Could you check a few things on this model? Use its own coordinates, in mm. Give positions to 0.01 mm unless a question says otherwise; leave off trailing zeros. Order: outer loops, then holes, each group sorted by start corner. A loop starts at its lowest first (then second) coordinate and runs counter-clockwise, first axis right, second up. Notation, with made-up numbers: M -22,4.25 L 37,4.25 A21 cw 37,29.25 Z; hole C -8,73 d2. An arc over 180 degrees is marked long. Return JSON: item names as keys, results as strings. Group by question number.
```python
from build123d import *

# Parameters (mm, degrees)
EXTRUDE_1_DEPTH            = 3.2
FILLET_1_R                 = 5
SKETCH_2_R                 = 2.1
CUT_EXTRUDE_1_DEPTH        = 3.2
PATTERN_LINEAR_1_COUNT     = 2
PATTERN_LINEAR_1_PITCH     = 45
PATTERN_LINEAR_1_COL_COUNT = 2
PATTERN_LINEAR_1_COL_PITCH = 45


with BuildPart() as part:
    # Эскиз1 → Бобышка-Вытянуть1 (new body)
    with BuildSketch(Plane.XY):
        Polygon((0, 0), (150, 0), (180, 220), (130, 220), align=None)
    extrude(amount=EXTRUDE_1_DEPTH)

    # Скругление1
    fillet_1_edges = [part.edges().sort_by_distance(p)[0] for p in [
        (130, 220, 1.6),
        (180, 220, 1.6),
        (150, 0, 1.6),
        (0, 0, 1.6),
    ]]
    fillet(fillet_1_edges, radius=FILLET_1_R)

    # Эскиз2 → Вырез-Вытянуть1 (cut)
    with BuildSketch(Plane.XY.offset(3.2)):
        with Locations((77.198893337, 10)):
            Circle(SKETCH_2_R)
    cut_extrude_1 = extrude(amount=-CUT_EXTRUDE_1_DEPTH, mode=Mode.SUBTRACT)

    # Линейный массив1: Вырез-Вытянуть1 ×2
    with Locations(*[(i * PATTERN_LINEAR_1_PITCH, 0, 0) for i in range(1, PATTERN_LINEAR_1_COUNT)]):
        add(cut_extrude_1, mode=Mode.SUBTRACT)

    # Линейный массив1 col: Вырез-Вытянуть1 ×2
    with Locations(*[(-i * PATTERN_LINEAR_1_COL_PITCH, 0, 0) for i in range(1, PATTERN_LINEAR_1_COL_COUNT)]):
        add(cut_extrude_1, mode=Mode.SUBTRACT)


solid = part.part
```
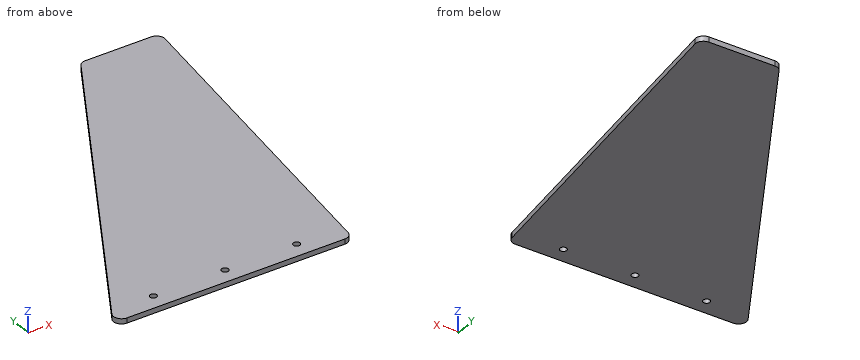
1. Imagine slicing it at A-A, the plane z = 1.8. Please give me the cut outline in (x, y), plus the area to 3 significant figures.
2. Imagine slicing it at B-B, the plane x = 65.5. Please give me the cut outline in (y, z), plus the area to 3 significant figures.
3. For pin 1 (2.5 mm diameter, centred on x = 77.2, y = 10, fed in from +Z); pin 2 (1 mm diameter, centred on x = 98, y = 57.5, fed in from -Z); pin 3 (1 mm diameter, centred on y = 144, z = 2, fed in from -X), each with a flat end and sliding along its axis, tell me the tip position at first contact or that it passes through.
4. Imagine slicing it at C-C, the plane y = 118. Please give me the cut outline in (x, z), plus the area to 3 significant figures.
5. I need wall thicknesses on L1, parallel to Y at x = 146, z = 0.9; L2, parallel to X at y = 138.5, z = 0.5; L3, parallel to Y at x = 53, z = 2.3. Which ranges of each line are inside material? Lowest first, please. Write a range as from..to.
Values:
{
 "1": {"outline": "M 4.46,7.54 A5 ccw 8.76,0 L 145.64,0 A5 ccw 150.59,4.32 L 179.23,214.32 A5 ccw 174.27,220 L 132.85,220 A5 ccw 128.55,217.54 Z; hole C 32.2,10 d4.2; hole C 77.2,10 d4.2; hole C 122.2,10 d4.2", "area": "21,900 mm²"},
 "2": {"outline": "M 0,0 L 110.85,0 L 110.85,3.2 L 0,3.2 Z", "area": "355 mm²"},
 "3": {"pin 1": "passes through", "pin 2": "stops at z = 0", "pin 3": "stops at x = 84.8"},
 "4": {"outline": "M 69.73,0 L 166.09,0 L 166.09,3.2 L 69.73,3.2 Z", "area": "308 mm²"},
 "5": {"L1": "y = 0.01..220", "L2": "x = 81.84..168.89", "L3": "y = 0..89.69"}
}
